Geometry check sheet. Reference: drawing and pictorial views, mm from the part's lowest x, y, z. Round coordinates to 2 decimals unless told otherwise and drop trailing zeros. Order: outer loops, then holes, each group sorted by start corner. A loop starts at its lowest first (then second) coordinate and runs counter-clockwise, first axis right, second up.
(1) Go/stop test with flat-tipped pins: pin 1 (12 mm diameter, centred on y = 9.5, z = 31.5, fed in from -X); pin 2 (6 mm diameter, centred on y = 9.5, z = 36, fed in from +X); pin 3 (3.5 mm diameter, centred on x = 38, z = 33.5, fed in from -Y). Record where each tip stops, or that it passes through.
(2) Material ranges on line 1 along Z through (x, y) = (38, 20.75); line 2 along Y through (x, z) = (1, 33); line 3 along Y through (x, z) = (40.5, 5), recorded low to high.
(3) Sectioned sample at D-D (z = 7). Record the boundary of the cut face in (x, y), plus the area to 3 significant figures.
(4) Release check for a two-part mould opening along X. For the marked faces 1, 2 and 3 record: +X half, -X half, draft (parallel to the pull), parting line (faces both ways), or undercut.
(5) Sectioned sample at A-A (z = 68.5). Record the boundary of the cut face in (x, y).
(6) Sectioned sample at C-C (x = 24). Record the boundary of the cut face in (y, z), plus the area to 3 significant figures.
(7) Sectioned sample at B-B (y = 12.5). Record the boundary of the cut face in (x, z), plus the area to 3 significant figures.
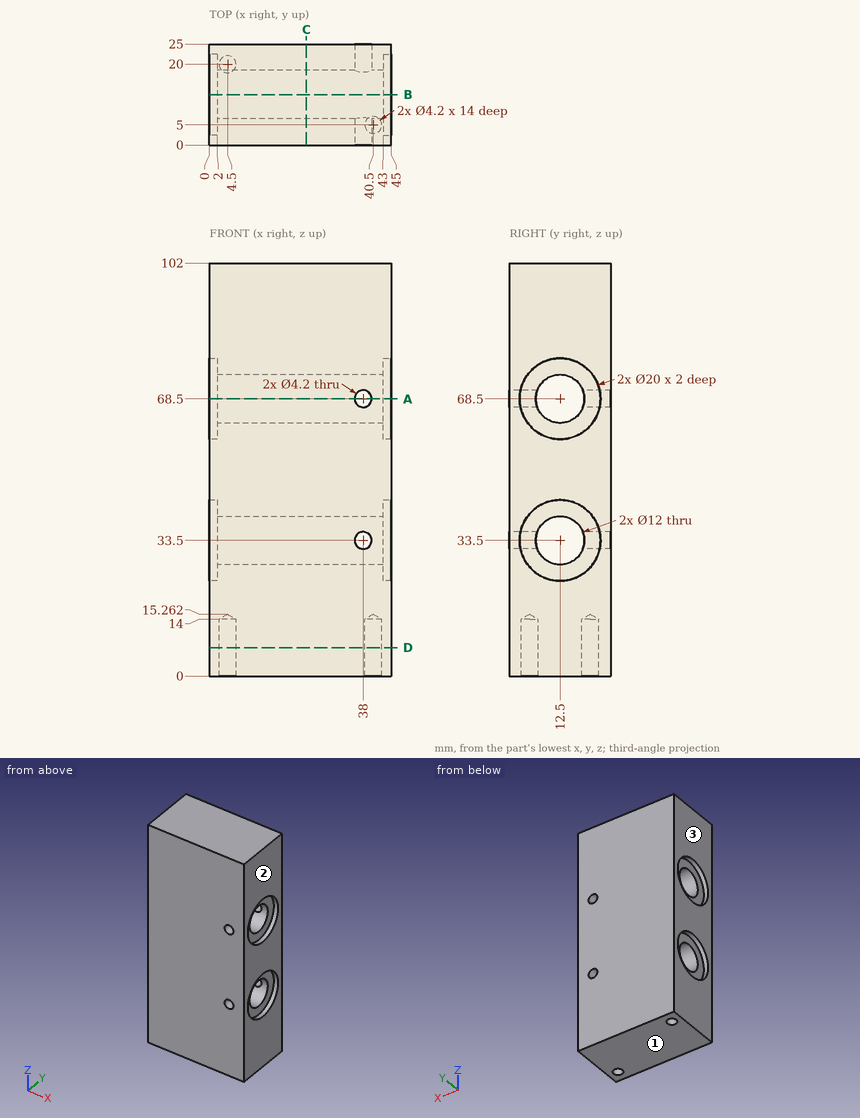
Answer below:
1. pin 1: stops at x = 2
1. pin 2: stops at x = 43
1. pin 3: passes through
2. line 1: z = 0 to 31.4, 35.6 to 66.4, 70.6 to 102
2. line 2: y = 0 to 2.51, 22.49 to 25
2. line 3: y = 0 to 2.9, 7.1 to 25
3. outline: (0, 0) - (45, 0) - (45, 25) - (0, 25) - close; hole circle Ø4.2 at (4.5, 20); hole circle Ø4.2 at (40.5, 5)
3. area: 1,100 mm2
4. face 1: draft
4. face 2: +X half
4. face 3: -X half
5. outline: (0, 0) - (35.9, 0) - (35.9, 6.5) - (2, 6.5) - (2, 2.5) - (0, 2.5) - close; (0, 22.5) - (2, 22.5) - (2, 18.5) - (35.9, 18.5) - (35.9, 25) - (0, 25) - close; (40.1, 0) - (45, 0) - (45, 2.5) - (43, 2.5) - (43, 6.5) - (40.1, 6.5) - close; (40.1, 18.5) - (43, 18.5) - (43, 22.5) - (45, 22.5) - (45, 25) - (40.1, 25) - close
6. outline: (0, 0) - (25, 0) - (25, 102) - (0, 102) - close; hole circle Ø12 at (12.5, 33.5); hole circle Ø12 at (12.5, 68.5)
6. area: 2,320 mm2
7. outline: (0, 0) - (45, 0) - (45, 23.5) - (43, 23.5) - (43, 27.5) - (2, 27.5) - (2, 23.5) - (0, 23.5) - close; (0, 43.5) - (2, 43.5) - (2, 39.5) - (43, 39.5) - (43, 43.5) - (45, 43.5) - (45, 58.5) - (43, 58.5) - (43, 62.5) - (2, 62.5) - (2, 58.5) - (0, 58.5) - close; (0, 78.5) - (2, 78.5) - (2, 74.5) - (43, 74.5) - (43, 78.5) - (45, 78.5) - (45, 102) - (0, 102) - close
7. area: 3,450 mm2
